Design review of the part built by this model. Coordinates are the model's own, in mm. Face numbers are marked on the shaded views. A direction names the side the tool comes from. Give positions to 0.01 mm unless a question says otherwise; leave off trailing zeros. Write each loop counter-clockwise with the first axis right and the second up, starting at its lowest first coordinate (ties: lowest second). Pieces come first, ordered by that corner, then holes. Notation, with made-up numbers: (-36, -12) -> (-32, -12) arc R28 cw to (-32, 25) -> close; hole circle Ø3 at (15, -17.5). An arc over 180 degrees is marked (long way). Answer as a JSON object with one key per item and string values.
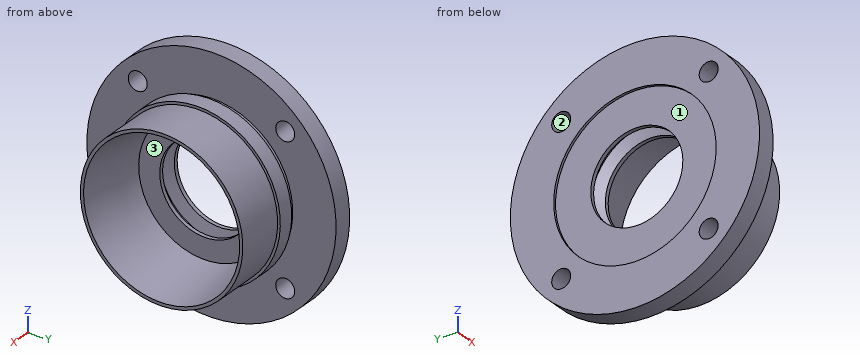
```python
from build123d import *

# Parameters (mm, degrees)
SKETCH_2_R          = 3.5
CUT_EXTRUDE_1_DEPTH = 74.218576878


with BuildPart() as part:
    # 草图1 → 旋转1 (revolve)
    with BuildSketch(Plane.XY, mode=Mode.PRIVATE) as revolve_1_sk:
        Polygon((3.6, 21.5), (2.5, 17), (1, 17), (1, 30), (0, 30), (0, 46), (7.2, 46), (7.2, 30), (9.2, 30), (9.2, 31), (15.2, 31), (15.2, 30), (33.6, 30), (33.6, 28.8226), (10.2, 24.78), (10.2, 17), (8.7, 17), (7.6, 21.5), align=None)
    revolve(revolve_1_sk.sketch.rotate(Axis((0, 0, 0), (1, 0, 0)), 90), axis=Axis((0, 0, 0), (1, 0, 0)))

    # 草图2 → 切除-拉伸1 (cut, through all)
    with BuildSketch(Plane.ZY):
        with Locations((-27.223611076, 27.223611076)):
            Circle(SKETCH_2_R)
        with Locations((27.223611076, 27.223611076)):
            Circle(SKETCH_2_R)
        with Locations((-27.223611076, -27.223611076)):
            Circle(SKETCH_2_R)
        with Locations((27.223611076, -27.223611076)):
            Circle(SKETCH_2_R)
    extrude(amount=-CUT_EXTRUDE_1_DEPTH, mode=Mode.SUBTRACT)


solid = part.part
```
(1) We need section C-C, the plane x = 14. State the section outline as (y, z) points, then the cut area to 3 significant figures.
Here are the results:
{"outline": "circle Ø62 at (0, 0); hole circle Ø50.87 at (0, 0)", "area": "986 mm²"}
(2) Clearance check with flat-ended pins moving along their axes: pin 1 (11 mm diameter, centred on y = -27.22, z = 27.22, fed in from +X); pin 2 (10 mm diameter, centred on x = 27, y = -4, fed in from -Z); pin 3 (6 mm diameter, centred on x = 4.5, z = 34.5, fed in from +Y). State where each tip first meets the part, or that it passes through.
Here are the results:
{"pin 1": "stops at x = 7.2", "pin 2": "stops at z = -30", "pin 3": "stops at y = 33.52"}
(3) For line 1 along Z through (x, y) = (2.5, 28); line 2 along Y through (x, z) = (0.75, 0); line 3 along X through (y, z) = (31.5, 3.5), list the stretches that pass through material, from the lowest coordinate up.
Here are the results:
{"line 1": "z = -36.5 to -30.64, -23.81 to 23.81, 30.64 to 36.5", "line 2": "y = -46 to -30, 30 to 46", "line 3": "x = 0 to 7.2"}
(4) We need section B-B, the plane z = 35.5. State the section outline as (x, y) points, then the cut area to 3 significant figures.
Here are the results:
{"outline": "(0, -29.25) -> (7.2, -29.25) -> (7.2, 29.25) -> (0, 29.25) -> close", "area": "421 mm²"}
(5) We need section A-A, the plane x = 5. State the section outline as (y, z) points, then the cut area to 3 significant figures.
Here are the results:
{"outline": "circle Ø92 at (0, 0); hole circle Ø7 at (-27.22, -27.22); hole circle Ø7 at (-27.22, 27.22); hole circle Ø43 at (0, 0); hole circle Ø7 at (27.22, -27.22); hole circle Ø7 at (27.22, 27.22)", "area": "5,040 mm²"}
(6) We need section D-D, the plane y = -36. State the section outline as (x, z) points.
Here are the results:
{"outline": "(0, -28.64) -> (7.2, -28.64) -> (7.2, 28.64) -> (0, 28.64) -> close"}
(7) For the marked faces 1, 2 and 3, list the 3-axis set-ups (+Z, -Z, +X, -X, +Y, -Y) from which the entire face can be reached by the end or side of a thin tool; tool diameter is ignored.
Here are the results:
{"face 1": "-X", "face 2": "+X, -X", "face 3": "+X"}
